Build history of the part. All positions in model axes, mm. Face numbers are marked on the shaded views. A direction names the side the tool comes from. Give positions to 0.01 mm unless a question says otherwise; leave off trailing zeros. Order: outer loops, then holes, each group sorted by start corner. A loop starts at its lowest first (then second) coordinate and runs counter-clockwise, first axis right, second up. Notation, with made-up numbers: (-17.5, 0.25) - (3.5, 0.25) arc R19 ccw to (3.5, 29.25) - close; hole circle Ø5 at (-31.5, -36.75). An arc over 180 degrees is marked (long way). Use a Markdown table: item, result.
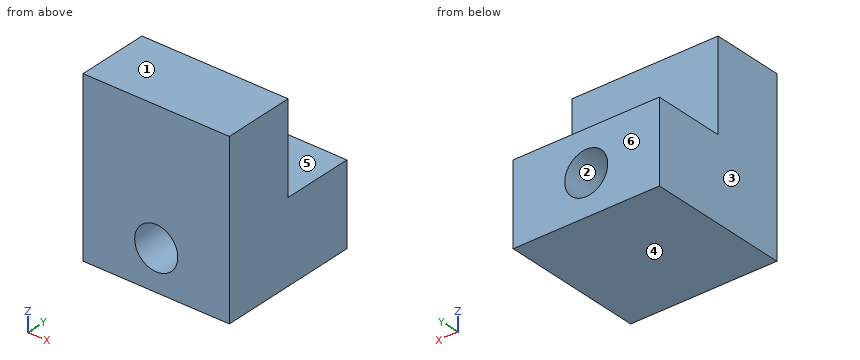
Autodesk Fusion 360 part; units mm, degrees
sketch "Sketch1" plane through (0, 0, 0) normal (0, 1, 0) x (1, 0, 0)
  line L0 (0, 0) -> (8.15, 0)
  line L1 (8.15, 0) -> (8.15, -4.5)
  line L2 (0, 0) -> (0, -4.5)
  line L3 (8.15, -4.5) -> (0, -4.5)
  line L4 (4.075, 0) -> (4.075, -4.5)
  circle A0 centre (4.075, -2.25) radius 1.75
  dimension "d1" = 8.15
  dimension "d2" = 4.5
  dimension "d3" = 4.5
  dimension "d4" = 3.5
extrude "Extrude1" add sketch "Sketch1" along normal blind 8 contours L0 L2 L3 L4 A0 | L0 L1 L3 L4 A0
sketch "Sketch2" plane through (0, 0, 4.5) normal (0, 0, 1) x (1, 0, 0)
  line L0 (0, 0) -> (8.15, 0)
  line L1 (8.15, 0) -> (8.15, 8)
  line L2 (8.15, 8) -> (0, 8)
  line L3 (0, 8) -> (0, 0)
  line L4 (0, 8) -> (0, 3.5)
  line L5 (0, 3.5) -> (0, 0)
  line L6 (0, 4) -> (8.15, 4)
  line L7 (8.15, 4) -> (8.15, 0)
  line L8 (8.15, 0) -> (0, 0)
  dimension "d7" = 4.5
extrude "Extrude2" add sketch "Sketch2" along normal blind 5 contours L0 L1 L3 L4 L5 L6 L7 L8
sketch "Sketch3" plane through (0, 8, 0) normal (0, 1, 0) x (-1, 0, 0)
  circle A0 centre (-4.075, 2.25) radius 1.75
  line L0 (0, 0) -> (0, 4.5)
  line L1 (0, 4.5) -> (-8.15, 4.5)
  line L2 (-8.15, 4.5) -> (-8.15, 0)
  line L3 (-8.15, 0) -> (0, 0)
  circle A1 centre (-4.075, 2.25) radius 1
  dimension "d10" = 2
extrude "Extrude3" add sketch "Sketch3" against normal blind 8 contours A0
sketch "Sketch4" plane through (0, 8, 0) normal (0, 1, 0) x (-1, 0, 0)
  circle A0 centre (-4.075, 2.25) radius 1
  line L0 (0, 0) -> (0, 4.5)
  line L1 (0, 4.5) -> (-8.15, 4.5)
  line L2 (-8.15, 4.5) -> (-8.15, 0)
  line L3 (-8.15, 0) -> (0, 0)
  circle A1 centre (-4.075, 2.25) radius 0.75
  dimension "d13" = 1.5
extrude "Extrude4" add sketch "Sketch4" against normal blind 8 contours A0
sketch "Sketch5" plane through (0, 8, 0) normal (0, 1, 0) x (-1, 0, 0)
  circle A0 centre (-4.075, 2.25) radius 0.75
  line L0 (0, 0) -> (0, 4.5)
  line L1 (0, 4.5) -> (-8.15, 4.5)
  line L2 (-8.15, 4.5) -> (-8.15, 0)
  line L3 (-8.15, 0) -> (0, 0)
  circle A1 centre (-4.075, 2.25) radius 1.2
  dimension "d17" = 2.4
extrude "Extrude5" cut sketch "Sketch5" against normal blind 20 contours A1
equation "HoleDiameter = 2 mm"
1) Wall check: line 1 (Z direction, x = 4, y = 1); line 2 (Z direction, x = 6.25, y = 7); line 3 (Z direction, x = 4.75, y = 0.75). Give the ranges that are in metal, low to high. Write a range as from..to.
Computed:
| item | result |
|---|---|
| line 1 | z = 0..1.05, 3.45..9.5 |
| line 2 | z = 0..4.5 |
| line 3 | z = 0..1.26, 3.24..9.5 |
2) Slice it at D-D (y = 3). Write the cut outline in (x, z) (3 decimals).
Computed:
| item | result |
|---|---|
| outline | (0, 0) - (8.15, 0) - (8.15, 9.5) - (0, 9.5) - close; hole circle Ø2.4 at (4.075, 2.25) |
3) Pin check, flat tips, straight feed: P1, Ø2, axis at x = 5, y = 5.5, coming from the +Z side; P2, Ø4, axis at x = 1.5, z = 5.5, coming from the -Y side; P3, Ø1.5, axis at x = 3.5, z = 6.5, coming from the +Y side. Stop position of each tip, or through.
Computed:
| item | result |
|---|---|
| P1 | stops at z = 4.5 |
| P2 | stops at y = 0 |
| P3 | stops at y = 4 |
4) Two-plate mould, pull along Z, no slides. Class the marked faces 1, 2, 3 and 4: +Z half, -Z half, draft (parallel to the pull), parting line (faces both ways), or undercut.
Computed:
| item | result |
|---|---|
| face 1 | +Z half |
| face 2 | undercut |
| face 3 | draft |
| face 4 | -Z half |
5) Tool access for the marked faces 5 and 6: list every direction of +Z, -Z, +X, -X, +Y, -Y with a clear straight run to the whole face (end or side of a thin tool).
Computed:
| item | result |
|---|---|
| face 5 | +Z, +X, -X, +Y |
| face 6 | +Z, -Z, +X, -X, +Y |
6) Slice it at C-C (x = 6). Write the cut outline in (y, z), and give its area (3 significant figures).
Computed:
| item | result |
|---|---|
| outline | (0, 0) - (8, 0) - (8, 4.5) - (4, 4.5) - (4, 9.5) - (0, 9.5) - close |
| area | 56.0 mm² |
7) Slice it at A-A (z = 2.25). Write the cut outline in (x, y) (3 decimals), and give its area (3 significant figures).
Computed:
| item | result |
|---|---|
| outline | (0, 0) - (2.875, 0) - (2.875, 8) - (0, 8) - close; (5.275, 0) - (8.15, 0) - (8.15, 8) - (5.275, 8) - close |
| area | 46.0 mm² |
8) Slice it at B-B (y = 4.25). Write the cut outline in (x, z) (3 decimals).
Computed:
| item | result |
|---|---|
| outline | (0, 0) - (8.15, 0) - (8.15, 4.5) - (0, 4.5) - close; hole circle Ø2.4 at (4.075, 2.25) |
